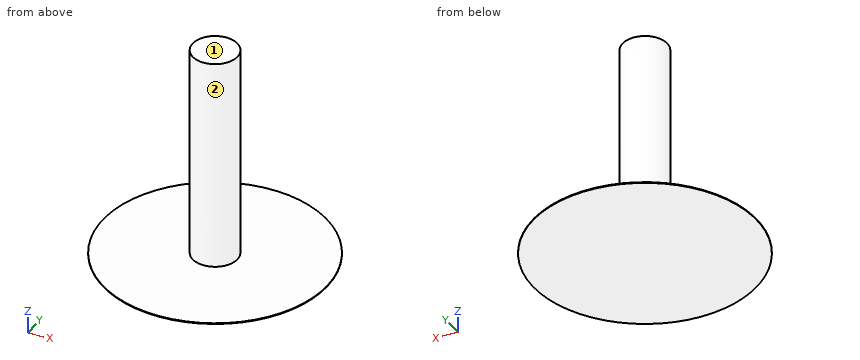
from build123d import *

# Parameters (mm, degrees)
CYLINDER_R        = 15
CYLINDER_DEPTH    = 10
CYLINDER001_R     = 3
CYLINDER001_DEPTH = 37.95
CYLINDER002_R     = 15
CYLINDER002_DEPTH = 0.1


with BuildPart() as cylinder:
    # Cylinder → Cylinder (new body)
    with BuildSketch(Plane.XY):
        Circle(CYLINDER_R)
    extrude(amount=CYLINDER_DEPTH)


with BuildPart() as cylinder001:
    # Cylinder001 → Cylinder001 (new body)
    with BuildSketch(Plane.XY.offset(-28.8499)):
        Circle(CYLINDER001_R)
    extrude(amount=CYLINDER001_DEPTH)


with BuildPart() as cut_spar:
    # Cylinder002 → Cylinder002 (new body)
    with BuildSketch(Plane.XY.offset(-28.9)):
        Circle(CYLINDER002_R)
    extrude(amount=CYLINDER002_DEPTH)

    # Fusion: union Cylinder001
    add(cylinder001.part)

    # Cut001: cut Cylinder
    add(cylinder.part, mode=Mode.SUBTRACT)


solid = cut_spar.part
Can you work these out from the model? Positions are in its coordinate system, mm. Face numbers are marked on the shaded views. A direction names the side the tool comes from. Give positions to 0.01 mm unless a question says otherwise; leave off trailing zeros. Write each loop counter-clockwise with the first axis right and the second up, starting at its lowest first coordinate (ties: lowest second). Pieces come first, ordered by that corner, then holes. Notation, with made-up numbers: M 79,-29 L 131,-29 A22 cw 131,-18 Z; hole C 50,13.5 d2. An arc over 180 degrees is marked long. Answer in a Markdown table with one row per item. Add a question column.
Item 1: Imagine slicing it at A-A, the plane x = 0. Write out the boundary of the cut face in (y, z).
Item 2: Imagine slicing it at C-C, the plane z = -16.25. Write out the boundary of the cut face in (x, y), plus the area to 3 significant figures.
Item 3: On a 3-axis mill with a long thin cutter (end or side, diameter ignored), from which of +Z, -Z, +X, -X, +Y, -Y can I reach the whole of each face in a straight line? I mean the marked faces 1 and 2. Say none if no direction works.
Item 4: Please list where these lines run through material, in increasing order: L1, parallel to X at y = 2, z = -24.5; L2, parallel to Y at x = -2.25, z = -20; L3, parallel to Y at x = -0.75, z = -14.75.
Item 5: For pin 1 Ø6 at (y, z) = (-1.5, -7.5) entering from -X; pin 2 Ø5 at (y, z) = (-9.5, -24.5) entering from -X; pin 3 Ø10 at (y, z) = (-3, -22.5) entering from +X; pin 4 Ø6 at (x, y) = (-7.5, -0.5) entering from +Z, each with a flat end and sliding along its axis, tell me the tip position at first contact or that it passes through.
Item 6: Imagine slicing it at D-D, the plane y = 11. Write out the boundary of the cut face in (x, z), plus the area to 3 significant figures.
Evaluation:
| question | item | result |
|---|---|---|
| 1 | outline | M -15,-28.9 L 15,-28.9 L 15,-28.8 L 3,-28.8 L 3,0 L -3,0 L -3,-28.8 L -15,-28.8 Z |
| 2 | outline | C 0,0 d6 |
| 2 | area | 28.3 mm² |
| 3 | face 1 | +Z, +X, -X, +Y, -Y |
| 3 | face 2 | +Z |
| 4 | L1 | x = -2.24 to 2.24 |
| 4 | L2 | y = -1.98 to 1.98 |
| 4 | L3 | y = -2.9 to 2.9 |
| 5 | pin 1 | stops at x = -3 |
| 5 | pin 2 | passes through |
| 5 | pin 3 | stops at x = 3 |
| 5 | pin 4 | stops at z = -28.8 |
| 6 | outline | M -10.2,-28.9 L 10.2,-28.9 L 10.2,-28.8 L -10.2,-28.8 Z |
| 6 | area | 2.04 mm² |
